```python
from build123d import *

# Parameters (mm, degrees)
F1_DEPTH = 12.7
F2_R     = 20.6375
F3_DEPTH = 29.3624
F4_T     = -1.5875
F5_R     = 0.79375
F6_R     = 2.38125
F7_R     = 2.38125


with BuildPart() as f1:
    # F0 (on Right) → F1 (new body)
    with BuildSketch(Plane.YZ):
        Polygon((4.7625, -2.749630657), (4.7625, 2.749630657), (0, 5.499261314), (-4.7625, 2.749630657), (-4.7625, -2.749630657), (0, -5.499261314), align=None)
    extrude(amount=F1_DEPTH)

    # F2 (on face) → F3 (join)
    with BuildSketch(Plane.YZ.offset(12.7)):
        Circle(F2_R)
    extrude(amount=F3_DEPTH)

    # F4
    f4_openings = [f1.faces().sort_by_distance(p)[0] for p in [
        (42.0624, 0, 0),
    ]]
    offset(amount=F4_T, openings=f4_openings, kind=Kind.INTERSECTION)

    # F5
    f5_edges = [f1.edges().sort_by_distance(p)[0] for p in [
        (14.2875, -19.05, 0),
    ]]
    fillet(f5_edges, radius=F5_R)

    # F6
    f6_edges = [f1.edges().sort_by_distance(p)[0] for p in [
        (12.7, -20.6375, 0),
    ]]
    fillet(f6_edges, radius=F6_R)

    # F7
    f7_edges = [f1.edges().sort_by_distance(p)[0] for p in [
        (0, 2.38125, 4.124446),
        (0, -2.38125, 4.124446),
        (0, -4.7625, 0),
        (0, -2.38125, -4.124446),
        (0, 2.38125, -4.124446),
        (0, 4.7625, 0),
    ]]
    fillet(f7_edges, radius=F7_R)


solid = f1.part
```
Geometry check sheet. Reference: the model listing, model coordinates, mm. A direction names the side the tool comes from. Give positions to 0.01 mm unless a question says otherwise; leave off trailing zeros. Write item = value, one per line. Start each with the question number.
1. Thickness scan on probe 1 along Z at (x, y) = (32, 0); probe 2 along Z at (x, y) = (23.5, -14); probe 3 along X at (y, z) = (-14, 10). Record the ranges inside material, lowest first.
2. Draft check along Y on faces 1 (the face through (7.468, -2.348, 4.144)), 2 (the face through (28.383, -4.474, -20.147)), 3 (the face through (1.037, 2.14, 3.784)), 4 (the face through (1.588, 0, 0)). Enter one of: +Y half, -Y half, draft (parallel to the pull), parting line (faces both ways), or undercut.
3. Go/stop test with flat-tipped pins: P1, Ø18.5, axis at y = -7, z = -6, coming from the +X side; P2, Ø2, axis at x = 26, y = -15.5, coming from the -Z side; P3, Ø2.5, axis at x = 7.5, z = -0.5, coming from the +Y side; P4, Ø12, axis at x = 35.5, z = 0.5, coming from the -Y side. Record where each tip stops, or that it passes through.
4. Tool access check on faces 5 (the face through (7, -4.762, 0)), 6 (the face through (12.7, 4, -4)), 7 (the face through (7.849, 1.61, 2.737)), 8 (the face through (7.47, -2.41, -4.11)). Record the directions out of +Z, -Z, +X, -X, +Y, -Y that give a thin tool (end or side, any length) a straight path to the whole face; none if there is none.
Values follow:
q1.probe_1 = -20.64 to -19.05, 19.05 to 20.64
q1.probe_2 = -15.16 to -12.92, 12.92 to 15.16
q1.probe_3 = 12.7 to 14.29
q2.face_1 = -Y half
q2.face_2 = parting line
q2.face_3 = +Y half
q2.face_4 = undercut
q3.P1 = 14.32
q3.P2 = -14.69
q3.P3 = 4.76
q3.P4 = -20.64
q4.face_5 = +Z, -Z, -X, -Y
q4.face_6 = -X
q4.face_7 = +X
q4.face_8 = -Z, -X, -Y
